from build123d import *

# Parameters (mm, degrees)
BOSS_EXTRUDE1_DEPTH = 4
SKETCH2_R           = 4
BOSS_EXTRUDE2_DEPTH = 7
CHAMFER1_SIZE       = 1
SKETCH3_R           = 2.375
BOSS_EXTRUDE3_DEPTH = 3
SKETCH4_R           = 2
BOSS_EXTRUDE4_DEPTH = 10
FILLET2_R           = 3
FILLET3_R           = 1


with BuildPart() as part:
    # Sketch1 → Boss-Extrude1 (new body)
    with BuildSketch(Plane.XY):
        Polygon((8.248891971, 0), (4.124445986, 7.14375), (-4.124445986, 7.14375), (-8.248891971, 0), (-4.124445986, -7.14375), (4.124445986, -7.14375), align=None)
    extrude(amount=BOSS_EXTRUDE1_DEPTH)

    # Sketch2 → Boss-Extrude2 (add)
    with BuildSketch(Plane.XY.offset(4)):
        Circle(SKETCH2_R)
    extrude(amount=BOSS_EXTRUDE2_DEPTH)

    # Chamfer1
    chamfer1_edges = [part.edges().sort_by_distance(p)[0] for p in [
        (-4, 0, 11),
    ]]
    chamfer(chamfer1_edges, length=CHAMFER1_SIZE)

    # Sketch3 → Boss-Extrude3 (add)
    with BuildSketch(Plane(origin=(0, 0, 0), x_dir=(-1, 0, 0), z_dir=(0, 0, -1))):
        Circle(SKETCH3_R)
    extrude(amount=BOSS_EXTRUDE3_DEPTH)

    # Sketch4 → Boss-Extrude4 (add)
    with BuildSketch(Plane(origin=(0, 0, -3), x_dir=(-1, 0, 0), z_dir=(0, 0, -1))):
        Circle(SKETCH4_R)
    extrude(amount=BOSS_EXTRUDE4_DEPTH)

    # Fillet2
    fillet2_edges = [part.edges().sort_by_distance(p)[0] for p in [
        (4.124445986, -7.14375, 2),
        (-4.124445986, -7.14375, 2),
        (-8.248891971, 0, 2),
        (-4.124445986, 7.14375, 2),
        (4.124445986, 7.14375, 2),
        (8.248891971, 0, 2),
    ]]
    fillet(fillet2_edges, radius=FILLET2_R)

    # Fillet3
    fillet3_edges = [part.edges().sort_by_distance(p)[0] for p in [
        (2.375, 0, 0),
    ]]
    fillet(fillet3_edges, radius=FILLET3_R)


solid = part.part
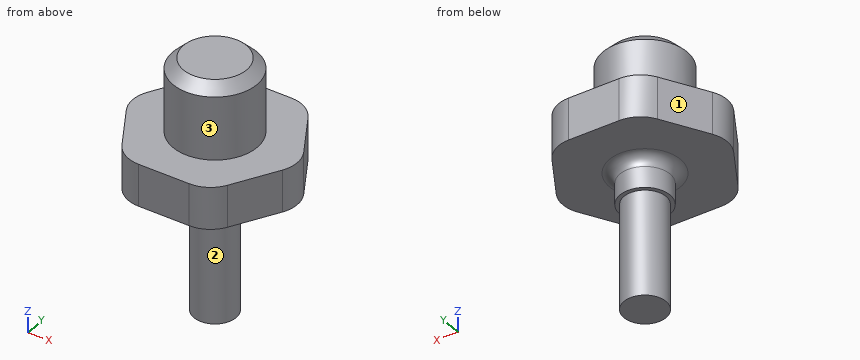
Verification items for the finished model (mm, model axes). Face numbers are marked on the shaded views. A direction names the side the tool comes from. Round coordinates to 2 decimals unless told otherwise and drop trailing zeros. Loops run counter-clockwise (first coordinate to the right, second up) from the corner with the lowest first, then second, coordinate; pieces in that order, holes last. Notation, with made-up numbers: M 8,-23.5 L 33,-23.5 A36 cw 33,13.5 Z; hole C 38,47 d10. An arc over 180 degrees is marked long. Write each question's results on one line, items separated by ' | '.
1) Gauge pin test, flat ends, axial feed: P1, Ø2, axis at x = -4, y = 4, coming from the +Z side; P2, Ø2, axis at x = 3, z = 7.5, coming from the +Y side; P3, Ø6, axis at y = 1.5, z = -5, coming from the +X side (3 decimals). Record the tip position at first contact, or that the pin passes through.
Checks:
P1: stops at z = 4 | P2: stops at y = 3.46 | P3: stops at x = 2.375
2) Access from +Z, -Z, +X, -X, +Y, -Y to the whole of each face (thin tool, end or side, straight path). Record for the marked faces 1, 2 and 3.
Checks:
face 1: +Z, -Z, -X, +Y | face 2: -Z | face 3: +Z
3) Section check D-D on z = -9.75. Record the boundary of the cut face in (x, y), then the cut area to 3 significant figures.
Checks:
outline: C 0,0 d4 | area: 12.6 mm2
4) Section check A-A on y = 0. Record the boundary of the cut face in (x, z) (3 decimals).
Checks:
outline: M -7.785,0 L -3.375,0 A1 cw -2.375,-1 L -2.375,-3 L -2,-3 L -2,-13 L 2,-13 L 2,-3 L 2.375,-3 L 2.375,-1 A1 cw 3.375,0 L 7.785,0 L 7.785,4 L 4,4 L 4,10 L 3,11 L -3,11 L -4,10 L -4,4 L -7.785,4 Z
5) Section check B-B on x = 0. Record the boundary of the cut face in (y, z) (3 decimals), then the cut area to 3 significant figures.
Checks:
outline: M -7.144,0 L -3.375,0 A1 cw -2.375,-1 L -2.375,-3 L -2,-3 L -2,-13 L 2,-13 L 2,-3 L 2.375,-3 L 2.375,-1 A1 cw 3.375,0 L 7.144,0 L 7.144,4 L 4,4 L 4,10 L 3,11 L -3,11 L -4,10 L -4,4 L -7.144,4 Z | area: 167 mm2
6) Section check C-C on z = 0.5. Record the boundary of the cut face in (x, y).
Checks:
outline: M -7.38,-1.5 L -4.99,-5.64 A3 ccw -2.39,-7.14 L 2.39,-7.14 A3 ccw 4.99,-5.64 L 7.38,-1.5 A3 ccw 7.38,1.5 L 4.99,5.64 A3 ccw 2.39,7.14 L -2.39,7.14 A3 ccw -4.99,5.64 L -7.38,1.5 A3 ccw Z
7) Scan lines: L1, parallel to Z at x = -4.5, y = -2.5; L2, parallel to X at y = 1.5, z = 3.75; L3, parallel to X at y = -2.5, z = 7. Record each from-to range of solid material in increasing order. Write a range as from..to.
Checks:
L1: z = 0..4 | L2: x = -7.38..7.38 | L3: x = -3.12..3.12
